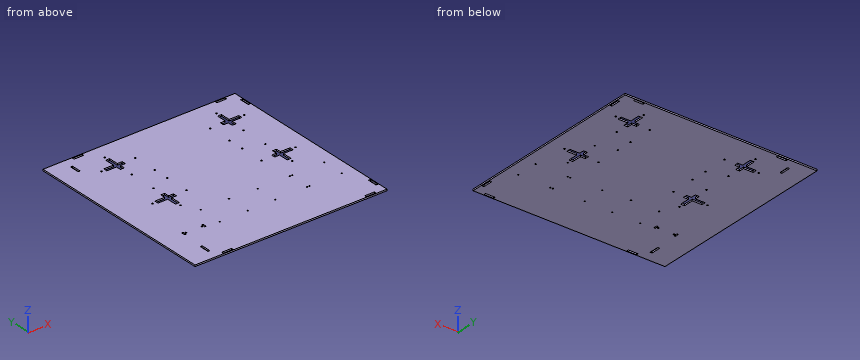
from build123d import *

# Parameters (mm, degrees)
SKETCH_W   = 395
SKETCH_H   = 395
SKETCH_R   = 1.25
SKETCH_R_2 = 1.5
SKETCH_W_2 = 20
SKETCH_H_2 = 4
SKETCH_W_3 = 4
SKETCH_H_3 = 20
SKETCH_W_4 = 3
SKETCH_H_4 = 8
PAD_DEPTH  = 3


with BuildPart() as part:
    # Sketch → Pad (new body)
    with BuildSketch(Plane.XY):
        Rectangle(SKETCH_W, SKETCH_H)
        with Locations((-21.5, -63.5)):
            Circle(SKETCH_R, mode=Mode.SUBTRACT)
        with Locations((-21.5, -112.5)):
            Circle(SKETCH_R, mode=Mode.SUBTRACT)
        with Locations((-58, 133.5)):
            Circle(SKETCH_R_2, mode=Mode.SUBTRACT)
        with Locations((96, 133.5)):
            Circle(SKETCH_R_2, mode=Mode.SUBTRACT)
        with Locations((-58, 0.5)):
            Circle(SKETCH_R_2, mode=Mode.SUBTRACT)
        with Locations((96, 0.5)):
            Circle(SKETCH_R_2, mode=Mode.SUBTRACT)
        with Locations((-58, 83.5)):
            Circle(SKETCH_R_2, mode=Mode.SUBTRACT)
        with Locations((-58, 50.5)):
            Circle(SKETCH_R_2, mode=Mode.SUBTRACT)
        with Locations((96, 83.5)):
            Circle(SKETCH_R_2, mode=Mode.SUBTRACT)
        with Locations((96, 50.5)):
            Circle(SKETCH_R_2, mode=Mode.SUBTRACT)
        with Locations((-128, 133.5)):
            Circle(SKETCH_R_2, mode=Mode.SUBTRACT)
        with Locations((-96, 165.5)):
            Circle(SKETCH_R_2, mode=Mode.SUBTRACT)
        with Locations((-96, 95.5)):
            Circle(SKETCH_R_2, mode=Mode.SUBTRACT)
        with Locations((-96, 38.5)):
            Circle(SKETCH_R_2, mode=Mode.SUBTRACT)
        with Locations((-128, 0.5)):
            Circle(SKETCH_R_2, mode=Mode.SUBTRACT)
        with Locations((-96, -31.5)):
            Circle(SKETCH_R_2, mode=Mode.SUBTRACT)
        with Locations((134, -31.5)):
            Circle(SKETCH_R_2, mode=Mode.SUBTRACT)
        with Locations((166, 0.5)):
            Circle(SKETCH_R_2, mode=Mode.SUBTRACT)
        with Locations((134, 38.5)):
            Circle(SKETCH_R_2, mode=Mode.SUBTRACT)
        with Locations((134, 95.5)):
            Circle(SKETCH_R_2, mode=Mode.SUBTRACT)
        with Locations((166, 133.5)):
            Circle(SKETCH_R_2, mode=Mode.SUBTRACT)
        with Locations((134, 165.5)):
            Circle(SKETCH_R_2, mode=Mode.SUBTRACT)
        with Locations((35, -67)):
            Circle(SKETCH_R, mode=Mode.SUBTRACT)
        with Locations((35, -112)):
            Circle(SKETCH_R, mode=Mode.SUBTRACT)
        with Locations((101, -67)):
            Circle(SKETCH_R, mode=Mode.SUBTRACT)
        with Locations((106, -67)):
            Circle(SKETCH_R, mode=Mode.SUBTRACT)
        with Locations((172, -67)):
            Circle(SKETCH_R, mode=Mode.SUBTRACT)
        with Locations((172, -112)):
            Circle(SKETCH_R, mode=Mode.SUBTRACT)
        with Locations((106, -112)):
            Circle(SKETCH_R, mode=Mode.SUBTRACT)
        with Locations((101, -112)):
            Circle(SKETCH_R, mode=Mode.SUBTRACT)
        with Locations((-79.5, -63.5)):
            Circle(SKETCH_R, mode=Mode.SUBTRACT)
        with Locations((-79.5, -112.5)):
            Circle(SKETCH_R, mode=Mode.SUBTRACT)
        with Locations((-144.2, -106.5)):
            Circle(SKETCH_R_2, mode=Mode.SUBTRACT)
        with Locations((-111.3, -106.5)):
            Circle(SKETCH_R_2, mode=Mode.SUBTRACT)
        Polygon((-100, 157.5), (-92, 157.5), (-92, 137.5), (-82, 137.5), (-82, 129.5), (-92, 129.5), (-92, 119.5), (-100, 119.5), (-100, 129.5), (-120, 129.5), (-120, 137.5), (-100, 137.5), align=None, mode=Mode.SUBTRACT)
        Polygon((120, 137.5), (130, 137.5), (130, 157.5), (138, 157.5), (138, 137.5), (158, 137.5), (158, 129.5), (138, 129.5), (138, 119.5), (130, 119.5), (130, 129.5), (120, 129.5), align=None, mode=Mode.SUBTRACT)
        Polygon((-100, 14.5), (-92, 14.5), (-92, 4.5), (-82, 4.5), (-82, -3.5), (-92, -3.5), (-92, -23.5), (-100, -23.5), (-100, -3.5), (-120, -3.5), (-120, 4.5), (-100, 4.5), align=None, mode=Mode.SUBTRACT)
        Polygon((130, 14.5), (138, 14.5), (138, 4.5), (158, 4.5), (158, -3.5), (138, -3.5), (138, -23.5), (130, -23.5), (130, -3.5), (120, -3.5), (120, 4.5), (130, 4.5), align=None, mode=Mode.SUBTRACT)
        with Locations((166, 194)):
            Rectangle(SKETCH_W_2, SKETCH_H_2, mode=Mode.SUBTRACT)
        with Locations((194, 166)):
            Rectangle(SKETCH_W_3, SKETCH_H_3, mode=Mode.SUBTRACT)
        with Locations((-128, 194)):
            Rectangle(SKETCH_W_2, SKETCH_H_2, mode=Mode.SUBTRACT)
        with Locations((-156, 166)):
            Rectangle(SKETCH_W_3, SKETCH_H_3, mode=Mode.SUBTRACT)
        with Locations((-152, -166)):
            Rectangle(SKETCH_W_3, SKETCH_H_3, mode=Mode.SUBTRACT)
        with Locations((-128, -194)):
            Rectangle(SKETCH_W_2, SKETCH_H_2, mode=Mode.SUBTRACT)
        with Locations((166, -194)):
            Rectangle(SKETCH_W_2, SKETCH_H_2, mode=Mode.SUBTRACT)
        with Locations((194, -166)):
            Rectangle(SKETCH_W_3, SKETCH_H_3, mode=Mode.SUBTRACT)
        with Locations((-107, -106.5)):
            Rectangle(SKETCH_W_4, SKETCH_H_4, mode=Mode.SUBTRACT)
        with Locations((-148.5, -106.5)):
            Rectangle(SKETCH_W_4, SKETCH_H_4, mode=Mode.SUBTRACT)
    extrude(amount=PAD_DEPTH)


with BuildPart() as part_1:
    # Body placement: moved
    add(part.part.moved(Location((200, -200, 0))))


solid = part_1.part
Could you check a few things on this model? Use its own coordinates, in mm. Coordinates: 2 decimals unless noted, no trailing zeros. Order: outer loops, then holes, each group sorted by start corner. A loop starts at its lowest first (then second) coordinate and runs counter-clockwise, first axis right, second up. Notation, with made-up numbers: (74, 69) -> (130, 69) arc R34 cw to (130, 105) -> close; hole circle Ø1 at (-25, 44). An arc over 180 degrees is marked (long way). One line per question, with ' | ' between items.
Q1. Imagine slicing it at A-A on y = -219. Please give me the cut outline in (x, z), and give its area (3 significant figures).
Return value:
outline: (2.5, 0) -> (100, 0) -> (100, 3) -> (2.5, 3) -> close; (108, 0) -> (330, 0) -> (330, 3) -> (108, 3) -> close; (338, 0) -> (397.5, 0) -> (397.5, 3) -> (338, 3) -> close | area: 1,140 mm²
Q2. Imagine slicing it at C-C on z = 2.35. State how many separate pieces and enclosed holes the cut face has, and give its area (3 significant figures).
Return value:
separate pieces: 1 | enclosed holes: 48 | area: 153,000 mm²
Q3. If I drill on L1, parallel to X at y = -31.5, z = 2.85; L2, parallel to Y at x = 354, z = 0.2; L3, parallel to X at y = -116.5, z = 2.35, over which ranges is the centre line in solid material (lowest first)?
Return value:
L1: 2.5 to 42, 46 to 392, 396 to 397.5 | L2: -397.5 to -203.5, -195.5 to -70.5, -62.5 to -2.5 | L3: 2.5 to 140.5, 143.5 to 294.5, 297.5 to 397.5
Q4. Imagine slicing it at B-B on x = 351. Please give me the cut outline in (y, z), and give its area (3 significant figures).
Return value:
outline: (-397.5, 0) -> (-203.5, 0) -> (-203.5, 3) -> (-397.5, 3) -> close; (-195.5, 0) -> (-70.5, 0) -> (-70.5, 3) -> (-195.5, 3) -> close; (-62.5, 0) -> (-2.5, 0) -> (-2.5, 3) -> (-62.5, 3) -> close | area: 1,140 mm²
Q5. I'm going to push a flat-ended pin straight in: P1, Ø3.5, axis at x = 104, y = -161.5, coming from the -Z side. Where does the tip first touch, or does it pass through?
Return value:
P1: z = 0
